```python
from build123d import *

# Parameters (mm, degrees)
SKETCH2_W               = 311
SKETCH2_H               = 135
BOSS_EXTRUDE1_DEPTH     = 10
BOSS_EXTRUDE2_DEPTH     = 311
FILLET1_R               = 10
FILLET2_R               = 5
CUT_EXTRUDE_THIN1_DEPTH = 0.5
CUT_EXTRUDE1_DEPTH      = 3
SKETCH8_R               = 6
BOSS_EXTRUDE3_DEPTH     = 10
BOSS_EXTRUDE3_TAPER     = 4


with BuildPart() as part:
    # Sketch2 → Boss-Extrude1 (new body)
    with BuildSketch(Plane(origin=(0, 0, 0), x_dir=(1, 0, 0), z_dir=(0, 0.9781476007338056, 0.2079116908177598))):
        with Locations((155.5, 67.5)):
            Rectangle(SKETCH2_W, SKETCH2_H)
    extrude(amount=-BOSS_EXTRUDE1_DEPTH)

    # Sketch5 → Boss-Extrude2 (add)
    with BuildSketch(Plane.ZY):
        Polygon((-134.129043007, 18.286602253), (-132.399185443, 9.762104074), (-2.079116908, -9.781476007), align=None)
    extrude(amount=-BOSS_EXTRUDE2_DEPTH)

    # Fillet1
    fillet1_edges = [part.edges().sort_by_distance(p)[0] for p in [
        (155.5, 18.286602253, -134.129043007),
    ]]
    fillet(fillet1_edges, radius=FILLET1_R)

    # Fillet2
    fillet2_edges = [part.edges().sort_by_distance(p)[0] for p in [
        (311, 24.193330233, -132.873529217),
        (0, 24.193330233, -132.873529217),
        (0, 13.006413151, -133.057545909),
        (0, 18.285616937, -133.915549829),
        (311, 13.006413151, -133.057545909),
        (311, 18.285616937, -133.915549829),
        (311, -4.890738004, -1.039558454),
        (0, -4.890738004, -1.039558454),
    ]]
    fillet(fillet2_edges, radius=FILLET2_R)

    # Sketch6 → Cut-Extrude-Thin1 (cut)
    # profile 1 of 2: a face of its own
    with BuildSketch(Plane(origin=(0, 0, 0), x_dir=(1, 0, 0), z_dir=(0, 0.9781476007338056, 0.20791169081775976))):
        with BuildLine():
            Line((3, 120), (3, 8))
            ThreePointArc((3, 8), (4.464466094, 4.464466094), (8, 3))
            Line((8, 3), (303, 3))
            ThreePointArc((303, 3), (306.535533906, 4.464466094), (308, 8))
            Line((308, 8), (308, 120))
            ThreePointArc((308, 120), (306.535533906, 123.535533906), (303, 125))
            Line((303, 125), (8, 125))
            ThreePointArc((8, 125), (4.464466094, 123.535533906), (3, 120))
        make_face()
        with BuildLine():
            Line((3.5, 120), (3.5, 8))
            ThreePointArc((3.5, 8), (4.818019485, 4.818019485), (8, 3.5))
            Line((8, 3.5), (303, 3.5))
            ThreePointArc((303, 3.5), (306.181980515, 4.818019485), (307.5, 8))
            Line((307.5, 8), (307.5, 120))
            ThreePointArc((307.5, 120), (306.181980515, 123.181980515), (303, 124.5))
            Line((303, 124.5), (8, 124.5))
            ThreePointArc((8, 124.5), (4.818019485, 123.181980515), (3.5, 120))
        make_face(mode=Mode.SUBTRACT)
    # profile 2 of 2: a face of its own
    with BuildSketch(Plane(origin=(0, 0, 0), x_dir=(1, 0, 0), z_dir=(0, 0.9781476007338056, 0.20791169081775976))):
        with BuildLine():
            ThreePointArc((15, 10), (11.464466094, 11.464466094), (10, 15))
            Line((10, 15), (9.5, 15))
            ThreePointArc((9.5, 15), (11.110912703, 11.110912703), (15, 9.5))
            Line((15, 9.5), (15, 10))
        make_face()
    extrude(amount=-CUT_EXTRUDE_THIN1_DEPTH, mode=Mode.SUBTRACT)

    # Sketch7 → Cut-Extrude1 (cut)
    with BuildSketch(Plane(origin=(0, 0, 0), x_dir=(1, 0, 0), z_dir=(0, 0.9781476007338056, 0.20791169081775976))):
        with BuildLine():
            Line((9, 119), (20.6, 119))
            ThreePointArc((20.6, 119), (22.014213562, 118.414213562), (22.6, 117))
            Line((22.6, 117), (22.6, 104.3))
            ThreePointArc((22.6, 104.3), (22.014213562, 102.885786438), (20.6, 102.3))
            Line((20.6, 102.3), (9, 102.3))
            ThreePointArc((9, 102.3), (7.585786438, 102.885786438), (7, 104.3))
            Line((7, 104.3), (7, 117))
            ThreePointArc((7, 117), (7.585786438, 118.414213562), (9, 119))
        make_face()
        with BuildLine():
            Line((302.6, 24.05), (290.675, 24.05))
            ThreePointArc((290.675, 24.05), (289.260786438, 24.635786438), (288.675, 26.05))
            Line((288.675, 26.05), (288.675, 38.8))
            ThreePointArc((288.675, 38.8), (288.089213562, 40.214213562), (286.675, 40.8))
            Line((286.675, 40.8), (275.025, 40.8))
            ThreePointArc((275.025, 40.8), (273.610786438, 40.214213562), (273.025, 38.8))
            Line((273.025, 38.8), (273.025, 26.05))
            ThreePointArc((273.025, 26.05), (272.439213562, 24.635786438), (271.025, 24.05))
            Line((271.025, 24.05), (259.1, 24.05))
            ThreePointArc((259.1, 24.05), (257.685786438, 23.464213562), (257.1, 22.05))
            Line((257.1, 22.05), (257.1, 9.3))
            ThreePointArc((257.1, 9.3), (257.685786438, 7.885786438), (259.1, 7.3))
            Line((259.1, 7.3), (302.6, 7.3))
            ThreePointArc((302.6, 7.3), (304.014213562, 7.885786438), (304.6, 9.3))
            Line((304.6, 9.3), (304.6, 22.05))
            ThreePointArc((304.6, 22.05), (304.014213562, 23.464213562), (302.6, 24.05))
        make_face()
        with BuildLine():
            Line((32.6, 119), (92.1, 119))
            ThreePointArc((92.1, 119), (93.514213562, 118.414213562), (94.1, 117))
            Line((94.1, 117), (94.1, 104.3))
            ThreePointArc((94.1, 104.3), (93.514213562, 102.885786438), (92.1, 102.3))
            Line((92.1, 102.3), (32.6, 102.3))
            ThreePointArc((32.6, 102.3), (31.185786438, 102.885786438), (30.6, 104.3))
            Line((30.6, 104.3), (30.6, 117))
            ThreePointArc((30.6, 117), (31.185786438, 118.414213562), (32.6, 119))
        make_face()
        with BuildLine():
            Line((99.1, 119), (158.6, 119))
            ThreePointArc((158.6, 119), (160.014213562, 118.414213562), (160.6, 117))
            Line((160.6, 117), (160.6, 104.3))
            ThreePointArc((160.6, 104.3), (160.014213562, 102.885786438), (158.6, 102.3))
            Line((158.6, 102.3), (99.1, 102.3))
            ThreePointArc((99.1, 102.3), (97.685786438, 102.885786438), (97.1, 104.3))
            Line((97.1, 104.3), (97.1, 117))
            ThreePointArc((97.1, 117), (97.685786438, 118.414213562), (99.1, 119))
        make_face()
        with BuildLine():
            Line((165.6, 119), (225.1, 119))
            ThreePointArc((225.1, 119), (226.514213562, 118.414213562), (227.1, 117))
            Line((227.1, 117), (227.1, 104.3))
            ThreePointArc((227.1, 104.3), (226.514213562, 102.885786438), (225.1, 102.3))
            Line((225.1, 102.3), (165.6, 102.3))
            ThreePointArc((165.6, 102.3), (164.185786438, 102.885786438), (163.6, 104.3))
            Line((163.6, 104.3), (163.6, 117))
            ThreePointArc((163.6, 117), (164.185786438, 118.414213562), (165.6, 119))
        make_face()
        with BuildLine():
            Line((232.1, 119), (275.6, 119))
            ThreePointArc((275.6, 119), (277.014213562, 118.414213562), (277.6, 117))
            Line((277.6, 117), (277.6, 104.3))
            ThreePointArc((277.6, 104.3), (277.014213562, 102.885786438), (275.6, 102.3))
            Line((275.6, 102.3), (232.1, 102.3))
            ThreePointArc((232.1, 102.3), (230.685786438, 102.885786438), (230.1, 104.3))
            Line((230.1, 104.3), (230.1, 117))
            ThreePointArc((230.1, 117), (230.685786438, 118.414213562), (232.1, 119))
        make_face()
        with BuildLine():
            Line((9, 95.3), (247.1, 95.3))
            ThreePointArc((247.1, 95.3), (248.514213562, 94.714213562), (249.1, 93.3))
            Line((249.1, 93.3), (249.1, 9.3))
            ThreePointArc((249.1, 9.3), (248.514213562, 7.885786438), (247.1, 7.3))
            Line((247.1, 7.3), (9, 7.3))
            ThreePointArc((9, 7.3), (7.585786438, 7.885786438), (7, 9.3))
            Line((7, 9.3), (7, 93.3))
            ThreePointArc((7, 93.3), (7.585786438, 94.714213562), (9, 95.3))
        make_face()
        with BuildLine():
            Line((259.1, 95.3), (302.6, 95.3))
            ThreePointArc((302.6, 95.3), (304.014213562, 94.714213562), (304.6, 93.3))
            Line((304.6, 93.3), (304.6, 63.8))
            ThreePointArc((304.6, 63.8), (304.014213562, 62.385786438), (302.6, 61.8))
            Line((302.6, 61.8), (259.1, 61.8))
            ThreePointArc((259.1, 61.8), (257.685786438, 62.385786438), (257.1, 63.8))
            Line((257.1, 63.8), (257.1, 93.3))
            ThreePointArc((257.1, 93.3), (257.685786438, 94.714213562), (259.1, 95.3))
        make_face()
    extrude(amount=-CUT_EXTRUDE1_DEPTH, mode=Mode.SUBTRACT)

    # Sketch8 → Boss-Extrude3 (add)
    with BuildSketch(Plane(origin=(0, 0, 0), x_dir=(1, 0, 0), z_dir=(0, 0.9781476007338055, 0.20791169081775973))):
        with Locations((292.55, 110.65)):
            Circle(SKETCH8_R)
    extrude(amount=BOSS_EXTRUDE3_DEPTH, taper=BOSS_EXTRUDE3_TAPER)


solid = part.part
```
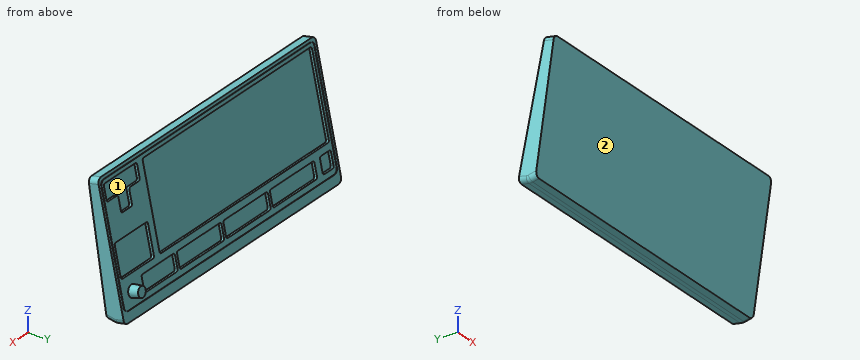
Source: CAD feature listing. Evaluate the final solid. Frame: model axes, mm. Face numbers are marked on the shaded views. Round coordinates to 2 decimals unless told otherwise and drop trailing zeros. Loops run counter-clockwise (first coordinate to the right, second up) from the corner with the lowest first, then second, coordinate; pieces in that order, holes last.
(1) Section query D-D (z = -55.5). Output: boundary loops of the cut face in (x, y).
From the geometry:
outline: (0, -1.77) - (311, -1.77) - (311, 11.8) - (308, 11.8) - (308, 11.29) - (307.5, 11.29) - (307.5, 11.8) - (249.1, 11.8) - (249.1, 8.73) - (7, 8.73) - (7, 11.8) - (3.5, 11.8) - (3.5, 11.29) - (3, 11.29) - (3, 11.8) - (0, 11.8) - close
(2) Contact query for flat-ended pins moving along their axis: pin 1 Ø2 at (x, y) = (62.5, -3) entering from +Z; pin 2 Ø12 at (x, y) = (153.5, 26) entering from -Z; pin 3 Ø2 at (x, z) = (154.5, -86) entering from +Y; pin 4 Ø1.7 at (y, z) = (22.5, -105.5) entering from +X. Output: stop coordinate, or through.
From the geometry:
pin 1: stops at z = -0.43
pin 2: stops at z = -133.76
pin 3: stops at y = 15.43
pin 4: stops at x = 311
(3) Section query C-C (z = -97). Output: boundary loops of the cut face in (x, y), and give its area (3 significant figures).
From the geometry:
outline: (0, 4.45) - (311, 4.45) - (311, 20.62) - (308, 20.62) - (308, 20.11) - (307.5, 20.11) - (307.5, 20.62) - (3.5, 20.62) - (3.5, 20.11) - (3, 20.11) - (3, 20.62) - (0, 20.62) - close
area: 5,030 mm2
(4) Pull-direction query (Z, two-part tool) for the marked faces 1 and 2; classes: +Z half, -Z half, draft (parallel to the pull), parting line (faces both ways), or undercut.
From the geometry:
face 1: undercut
face 2: -Z half
(5) Section query B-B (z = -75.5). Output: boundary loops of the cut face in (x, y), and give its area (3 significant figures).
From the geometry:
outline: (0, 1.23) - (311, 1.23) - (311, 16.05) - (308, 16.05) - (308, 15.54) - (307.5, 15.54) - (307.5, 16.05) - (304.6, 16.05) - (304.6, 12.98) - (257.1, 12.98) - (257.1, 16.05) - (249.1, 16.05) - (249.1, 12.98) - (7, 12.98) - (7, 16.05) - (3.5, 16.05) - (3.5, 15.54) - (3, 15.54) - (3, 16.05) - (0, 16.05) - close
area: 3,720 mm2
(6) Material intervals for probe 1 along Y at (x, z) = (273.5, -101); probe 2 along Y at (x, z) = (18, -109.5); probe 3 along X at (y, z) = (24, -108), sorted ascending.
From the geometry:
probe 1: y = 5.05 to 18.4
probe 2: y = 6.33 to 20.21
probe 3: x = 286.62 to 298.48
(7) Section query A-A (x = 117). Output: boundary loops of the cut face in (y, z) (1 decimal), and give its area (3 significant figures).
From the geometry:
outline: (-9.8, -2.1) - (9.8, -132.4) - (16.3, -133.7) arc R10 ccw to (20.3, -133.7) - (28.1, -132) - (26, -122.3) - (25.5, -122.4) - (25.4, -121.9) - (25.9, -121.8) - (24.7, -116.4) - (21.8, -117) - (18.3, -100.7) - (21.3, -100.1) - (19.8, -93.2) - (16.9, -93.8) - (-1.4, -7.8) - (1.5, -7.1) - (0.7, -3.4) - (0.2, -3.5) - (0.1, -3) - (0.6, -2.9) - (0, 0) - close
area: 1,570 mm2
